Could you check a few things on this drawing? It's one solid part, dimensions in mm from its lowest x, y, z. A direction names the side the tool comes from. Round coordinates to 2 decimals unless told otherwise and drop trailing zeros. Loops run counter-clockwise (first coordinate to the right, second up) from the corner with the lowest first, then second, coordinate; pieces in that order, holes last.
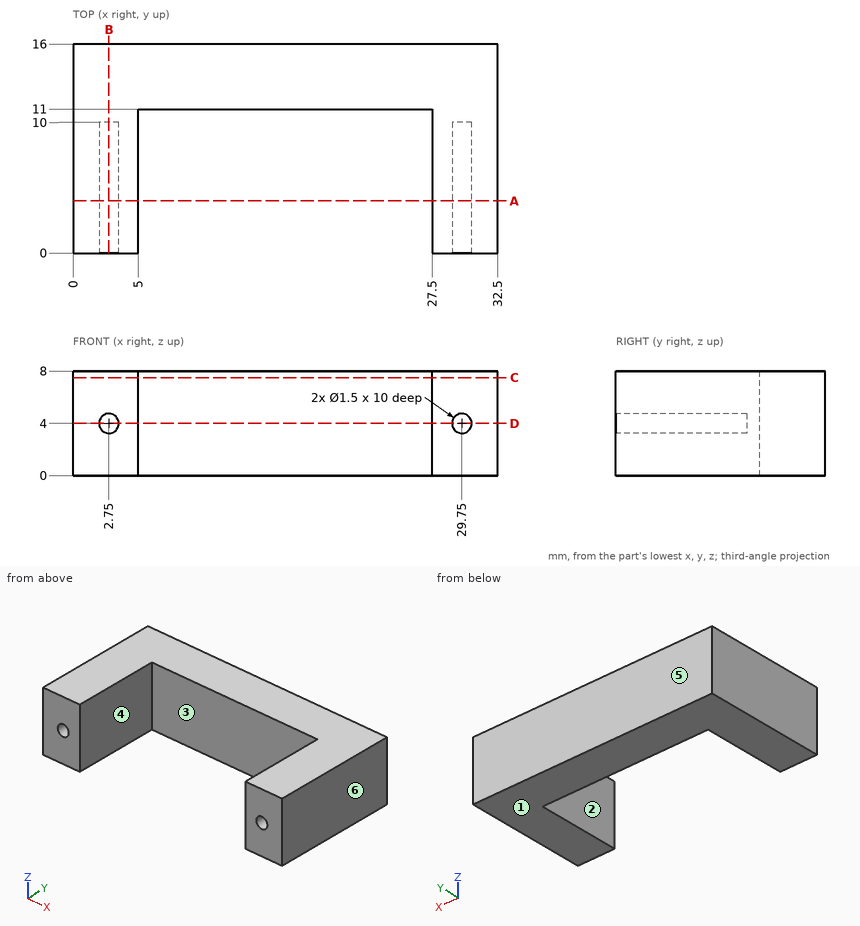
(1) If I drill on line 1 (X direction, y = 1.75, z = 0.5); line 2 (Z direction, x = 29.75, y = 6.5); line 3 (Y direction, x = 9, z = 3.5), over which ranges is the centre line in solid material (lowest first)?
(2) Which directions (+Z, -Z, +X, -X, +Y, -Y) give clear straight access to the entire face, cutting with the end or side of a thin tool? Please do the marked faces 1 and 2.
(3) Suppose I cut it at B-B (x = 2.75). Write out the boundary of the cut face in (y, z).
(4) For pin 1 (1.5 mm diameter, centred on y = 2.5, z = 5.5, fed in from -X); pin 2 (0.8 mm diameter, centred on x = 30, z = 4, fed in from -Y), each with a flat end and sliding along its axis, tell me the tip position at first contact or that it passes through.
(5) Suppose I cut it at A-A (y = 4). Write out the boundary of the cut face in (x, z), then the cut area to 3 significant figures.
(6) We'd pull the mould along X, two halves only. Please class the marked faces 3, 4, 5 and 6: released by +X, released by -X, zero draft, split by the parting line, or undercut.
(7) Suppose I cut it at C-C (z = 7.5). Write out the boundary of the cut face in (x, y), then the cut area to 4 significant figures.
(8) Suppose I cut it at D-D (z = 4). Write out the boundary of the cut face in (x, y), then the cut area to 4 significant figures.
Check result:
1. line 1: x = 0 to 5, 27.5 to 32.5
1. line 2: z = 0 to 3.25, 4.75 to 8
1. line 3: y = 11 to 16
2. face 1: -Z, +X, -X, +Y, -Y
2. face 2: +Z, -Z, -Y
3. outline: (0, 0) - (16, 0) - (16, 8) - (0, 8) - (0, 4.75) - (10, 4.75) - (10, 3.25) - (0, 3.25) - close
4. pin 1: stops at x = 0
4. pin 2: stops at y = 10
5. outline: (0, 0) - (5, 0) - (5, 8) - (0, 8) - close; (27.5, 0) - (32.5, 0) - (32.5, 8) - (27.5, 8) - close; hole circle Ø1.5 at (2.75, 4); hole circle Ø1.5 at (29.75, 4)
5. area: 76.5 mm2
6. face 3: undercut
6. face 4: undercut
6. face 5: zero draft
6. face 6: released by +X
7. outline: (0, 0) - (5, 0) - (5, 11) - (27.5, 11) - (27.5, 0) - (32.5, 0) - (32.5, 16) - (0, 16) - close
7. area: 272.5 mm2
8. outline: (0, 0) - (2, 0) - (2, 10) - (3.5, 10) - (3.5, 0) - (5, 0) - (5, 11) - (27.5, 11) - (27.5, 0) - (29, 0) - (29, 10) - (30.5, 10) - (30.5, 0) - (32.5, 0) - (32.5, 16) - (0, 16) - close
8. area: 242.5 mm2
